Here's how the part is built. I have some questions about the finished solid (model axes, mm). Face numbers are marked on the shaded views. Round coordinates to 2 decimals unless told otherwise and drop trailing zeros. Write each loop counter-clockwise with the first axis right and the second up, starting at its lowest first coordinate (ties: lowest second). Pieces come first, ordered by that corner, then holes. Notation, with made-up numbers: (45, -5.75) - (49, -5.75) arc R26 cw to (49, 29.25) - close; hole circle Ø7 at (37, 58). An arc over 180 degrees is marked (long way). One line per question, with ' | ' between items. Start each with the question number.
(1) Imagine slicing it at C-C (z = 90.5). Write out the boundary of the cut face in (x, y), plus the area to 3 significant figures.
(2) Will these pins go through, and if not, where does the flat tip stop? pin 1 (2.5 mm diameter, centred on x = -2, z = 2, fed in from -Y); pin 2 (4 mm diameter, centred on x = 12.5, y = 57, fed in from +Z); pin 3 (5 mm diameter, centred on x = -22, y = 77, fed in from -Z); pin 4 (2.5 mm diameter, centred on x = 7, z = 105.5, fed in from -Y).
(3) Imagine slicing it at D-D (x = -1). Write out the boundary of the cut face in (y, z).
(4) If I drill on L1, parallel to X at y = 48, z = 63; L2, parallel to Z at x = 9, y = -111.5; L3, parallel to Y at x = 68.5, z = 91.5, over which ranges is the centre line in solid material (lowest first)?
(5) Imagine slicing it at A-A (x = -54.5). Write out the boundary of the cut face in (y, z).
(6) Imagine slicing it at B-B (y = -20). Write out the boundary of the cut face in (x, z), plus the area to 3 significant figures.
(7) Thinking about a two-plate mould opening in X: for the marked faces 1, 2, 3 and 4, which applies, pulls with the +X half, pulls with the -X half, needs draft (parallel to the pull), parting line crosses it, or undercut?
from build123d import *

# Parameters (mm, degrees)
F0_W      = 165
F0_H      = 256
F0_W_2    = 159
F0_H_2    = 250
F1_DEPTH  = 100
F2_W      = 165
F2_H      = 256
F3_DEPTH  = 3
F4_W      = 165
F4_H      = 256
F5_DEPTH  = 3
F7_DEPTH  = 8
F9_DEPTH  = 8
F10_W     = 30
F10_H     = 65
F11_DEPTH = 2
F12_W     = 243
F12_H     = 8
F13_DEPTH = 3
F14_W     = 152
F14_H     = 8
F15_DEPTH = 3
F16_W     = 165
F16_H     = 15.5
F17_DEPTH = 3
F18_W     = 15.5
F18_H     = 240.5
F19_DEPTH = 3


with BuildPart() as f1:
    # F0 (on Top) → F1 (new body)
    with BuildSketch(Plane.XY):
        Rectangle(F0_W, F0_H)
        Rectangle(F0_W_2, F0_H_2, mode=Mode.SUBTRACT)
    extrude(amount=F1_DEPTH)

    # F2 (on face) → F3 (join)
    with BuildSketch(Plane.XY):
        Rectangle(F2_W, F2_H)
    extrude(amount=F3_DEPTH)

    # F4 (on face) → F5 (join)
    with BuildSketch(Plane.XY.offset(100)):
        Rectangle(F4_W, F4_H)
    extrude(amount=-F5_DEPTH)

    # F6 (on face) → F7 (join)
    with BuildSketch(Plane.XY.offset(100)):
        Polygon((-82.5, 128), (-82.5, -128), (-69.5, -128), (-69.5, 115), (82.5, 115), (82.5, 128), (-69.5, 128), (-73.5, 128), align=None)
    extrude(amount=F7_DEPTH)

    # F8 (on Top) → F9 (cut)
    with BuildSketch(Plane.XY):
        Polygon((-82.5, -128), (82.5, -128), (82.5, -115), (82.5, 128), (69.5, 128), (69.5, -115), (-82.5, -115), align=None)
    extrude(amount=F9_DEPTH, mode=Mode.SUBTRACT)

    # F10 (on face) → F11 (cut)
    with BuildSketch(Plane(origin=(0, 128, 0), x_dir=(-1, 0, 0), z_dir=(0, 1, 0))):
        with Locations((47.5, 32.5)):
            Rectangle(F10_W, F10_H)
    extrude(amount=-F11_DEPTH, mode=Mode.SUBTRACT)

    # F12 (on face) → F13 (join)
    with BuildSketch(Plane.YZ.offset(69.5)):
        with Locations((6.5, 4)):
            Rectangle(F12_W, F12_H)
    extrude(amount=-F13_DEPTH)

    # F14 (on face) → F15 (join)
    with BuildSketch(Plane.XZ.offset(115)):
        with Locations((-6.5, 4)):
            Rectangle(F14_W, F14_H)
    extrude(amount=-F15_DEPTH)

    # F16 (on face) → F17 (join)
    with BuildSketch(Plane(origin=(0, 0, 8), x_dir=(1, 0, 0), z_dir=(0, 0, -1))):
        with Locations((0, 120.25)):
            Rectangle(F16_W, F16_H)
    extrude(amount=-F17_DEPTH)

    # F18 (on face) → F19 (join)
    with BuildSketch(Plane(origin=(0, 0, 8), x_dir=(1, 0, 0), z_dir=(0, 0, -1))):
        with Locations((74.75, -7.75)):
            Rectangle(F18_W, F18_H)
    extrude(amount=-F19_DEPTH)


solid = f1.part
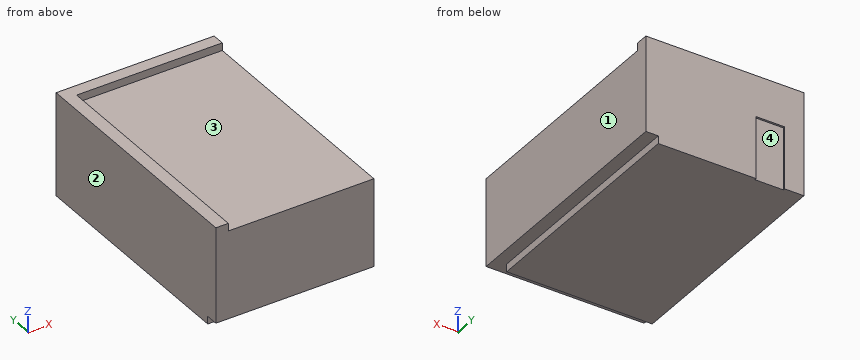
Check sheet entries:
1) outline: (-82.5, -128) - (82.5, -128) - (82.5, 128) - (-82.5, 128) - close; hole (-79.5, -125) - (79.5, -125) - (79.5, 125) - (-79.5, 125) - close | area: 2,490 mm^2
2) pin 1: y = -115 | pin 2: z = 100 | pin 3: z = 0 | pin 4: y = 115
3) outline: (-128, 8) - (-115, 8) - (-115, 0) - (128, 0) - (128, 108) - (115, 108) - (115, 100) - (-128, 100) - close; hole (-125, 11) - (-112.5, 11) - (-112.5, 8) - (-112, 8) - (-112, 3) - (125, 3) - (125, 97) - (-125, 97) - close
4) L1: -82.5 to -79.5, 79.5 to 82.5 | L2: 0 to 3, 97 to 100 | L3: -128 to -125, 125 to 128
5) outline: (-128, 8) - (-115, 8) - (-115, 0) - (126, 0) - (126, 65) - (128, 65) - (128, 108) - (115, 108) - (115, 100) - (-128, 100) - close; hole (-125, 11) - (-112.5, 11) - (-112.5, 8) - (-112, 8) - (-112, 3) - (125, 3) - (125, 97) - (-125, 97) - close
6) outline: (-82.5, 0) - (69.5, 0) - (69.5, 8) - (82.5, 8) - (82.5, 100) - (-69.5, 100) - (-69.5, 108) - (-82.5, 108) - close; hole (-79.5, 3) - (66.5, 3) - (66.5, 8) - (67, 8) - (67, 11) - (79.5, 11) - (79.5, 97) - (-79.5, 97) - close | area: 1,660 mm^2
7) face 1: pulls with the +X half | face 2: pulls with the -X half | face 3: needs draft | face 4: undercut
